Part model, mm, in its own coordinate system. A direction names the side the tool comes from. Coordinates: 2 decimals unless noted, no trailing zeros. Loops run counter-clockwise (first coordinate to the right, second up) from the corner with the lowest first, then second, coordinate; pieces in that order, holes last. Notation, with made-up numbers: (56, 82.5) -> (60, 82.5) arc R19 cw to (60, 97.5) -> close; hole circle Ø6 at (58.25, 31.25). An arc over 180 degrees is marked (long way). One line per item, written item: value. Start each with the question number.
from build123d import *

# Parameters (mm, degrees)
SKETCH4_R           = 1.5
BOSS_EXTRUDE1_DEPTH = 3.5
SKETCH6_R           = 2
CUT_EXTRUDE1_DEPTH  = 10


with BuildPart() as part:
    # Sketch4 → Boss-Extrude1 (new body)
    with BuildSketch(Plane.XY):
        with BuildLine():
            Line((59.884076231, 77.5), (62.057311876, 65.174968198))
            ThreePointArc((62.057311876, 65.174968198), (65, 62.232280074), (67.942688124, 65.174968198))
            Line((67.942688124, 65.174968198), (70.115923769, 77.5))
            Line((70.115923769, 77.5), (161.654067638, 77.5))
            Line((161.654067638, 77.5), (180, 92.5))
            Line((180, 92.5), (180, 107.5))
            Line((180, 107.5), (-50, 107.5))
            Line((-50, 107.5), (-50, 92.5))
            Line((-50, 92.5), (-30.115923769, 77.5))
            Line((-30.115923769, 77.5), (59.884076231, 77.5))
        make_face()
        with Locations((65, 65)):
            Circle(SKETCH4_R, mode=Mode.SUBTRACT)
        with BuildLine():
            Line((125, 82.5), (5, 82.5))
            ThreePointArc((5, 82.5), (-5, 92.5), (5, 102.5))
            Line((5, 102.5), (125, 102.5))
            ThreePointArc((125, 102.5), (135, 92.5), (125, 82.5))
        make_face(mode=Mode.SUBTRACT)
    extrude(amount=-BOSS_EXTRUDE1_DEPTH)

    # Sketch6 → Cut-Extrude1 (cut)
    with BuildSketch(Plane.XY):
        with Locations((-35, 102.5)):
            Circle(SKETCH6_R)
        with Locations((-35, 94.5)):
            Circle(SKETCH6_R)
        with Locations((165, 94.5)):
            Circle(SKETCH6_R)
        with Locations((165, 102.5)):
            Circle(SKETCH6_R)
    extrude(amount=-CUT_EXTRUDE1_DEPTH, mode=Mode.SUBTRACT)


solid = part.part
1) Slice it at C-C (z = -2.55). Give the cut face in (x, y).
2) Probe line 1 (Y direction, x = 65, z = -1.8); line 2 (X direction, y = 65, z = -1.8); line 3 (Y direction, x = -35, z = -2.6). List the from-to ranges inside material, lowest first. Write a range as from..to.
3) Slice it at D-D (x = -35). Give the cut face in (y, z).
4) Pin check, flat tips, straight feed: pin 1 Ø1.8 at (x, z) = (64, -1.5) entering from -Y; pin 2 Ø1.8 at (x, z) = (1.5, -1.5) entering from -Y; pin 3 Ø5 at (x, y) = (165, 94.5) entering from -Z; pin 4 Ø2.5 at (x, y) = (-35, 102.5) entering from +Z (3 decimals). Stop position of each tip, or through.
5) Slice it at B-B (y = 88). Give the cut face in (x, z), then the cut area to 3 significant figures.
6) Slice it at A-A (x = 80). Give the cut face in (y, z).
7) Tool access for faces 5 (the cylindrical face through (-5, 92.3, -1.7)), 6 (the flat face through (63, 80, -3.5)): list every direction of +Z, -Z, +X, -X, +Y, -Y with a clear straight run to the whole face (end or side of a thin tool).
8) Pull direction X, two halves, no side cores. Call faces 1 (the cylindrical face through (163.526, 95.852, -1.726)), 2 (the flat face through (63, 80, 0)), 3 (the flat face through (170.699, 84.895, -1.726)), 4 (the flat face through (-40.197, 85.105, -1.726)): +X half, -X half, draft (parallel to the pull), parting line (faces both ways), or undercut.
Check sheet entries:
1. outline: (-50, 92.5) -> (-30.12, 77.5) -> (59.88, 77.5) -> (62.06, 65.17) arc R2.94 ccw to (67.94, 65.17) -> (70.12, 77.5) -> (161.65, 77.5) -> (180, 92.5) -> (180, 107.5) -> (-50, 107.5) -> close; hole circle Ø4 at (-35, 94.5); hole circle Ø4 at (-35, 102.5); hole (5, 82.5) -> (125, 82.5) arc R10 ccw to (125, 102.5) -> (5, 102.5) arc R10 ccw to start; hole circle Ø3 at (65, 65); hole circle Ø4 at (165, 94.5); hole circle Ø4 at (165, 102.5)
2. line 1: y = 62.23..63.5, 66.5..82.5, 102.5..107.5
2. line 2: x = 62.06..63.5, 66.5..67.94
2. line 3: y = 81.18..92.5, 96.5..100.5, 104.5..107.5
3. outline: (81.18, -3.5) -> (92.5, -3.5) -> (92.5, 0) -> (81.18, 0) -> close; (96.5, -3.5) -> (100.5, -3.5) -> (100.5, 0) -> (96.5, 0) -> close; (104.5, -3.5) -> (107.5, -3.5) -> (107.5, 0) -> (104.5, 0) -> close
4. pin 1: stops at y = 62.23
4. pin 2: stops at y = 77.5
4. pin 3: stops at z = -3.5
4. pin 4: passes through
5. outline: (-44.03, -3.5) -> (-3.93, -3.5) -> (-3.93, 0) -> (-44.03, 0) -> close; (133.93, -3.5) -> (174.5, -3.5) -> (174.5, 0) -> (133.93, 0) -> close
5. area: 282 mm^2
6. outline: (77.5, -3.5) -> (82.5, -3.5) -> (82.5, 0) -> (77.5, 0) -> close; (102.5, -3.5) -> (107.5, -3.5) -> (107.5, 0) -> (102.5, 0) -> close
7. face 5: +Z, -Z
7. face 6: -Z, +X, -X, +Y, -Y
8. face 1: undercut
8. face 2: draft
8. face 3: +X half
8. face 4: -X half
